Part model, mm, in its own coordinate system. A direction names the side the tool comes from. Coordinates: 2 decimals unless noted, no trailing zeros. Order: outer loops, then holes, each group sorted by start corner. A loop starts at its lowest first (then second) coordinate and runs counter-clockwise, first axis right, second up.
```python
from build123d import *

# Parameters (mm, degrees)
SKETCH_1_R          = 1.6
SKETCH_1_R_2        = 2.1
EXTRUDE_1_DEPTH     = 20
EXTRUDE_2_DEPTH     = 20
SKETCH_3_R          = 1.6
CUT_EXTRUDE_1_DEPTH = 169.07736314
SKETCH_4_R          = 1.6
CUT_EXTRUDE_2_DEPTH = 169.07736314
SKETCH_6_W          = 50
SKETCH_6_H          = 15
SKETCH_6_W_2        = 77.817383139
SKETCH_6_H_2        = 81.542414759
CUT_EXTRUDE_3_DEPTH = 169.07736314
FILLET_1_R          = 2
CUT_EXTRUDE_4_DEPTH = 120.357877938
FILLET_2_R          = 1
SKETCH_8_W          = 15
SKETCH_8_H          = 22
SKETCH_8_H_2        = 25
CUT_EXTRUDE_5_DEPTH = 120.357877938
FILLET_3_R          = 10
FILLET_4_R          = 1
SKETCH_9_W          = 25.911411074
SKETCH_9_H          = 3
EXTRUDE_3_DEPTH     = 20
FILLET_5_R          = 1


with BuildPart() as part:
    # 草图1 → 凸台-拉伸1 (new body)
    with BuildSketch(Plane(origin=(0, 0, 0), x_dir=(1, 0, 0), z_dir=(0, 1, 0))):
        Polygon((-25, 0), (-19, 0), (-19, 165), (19, 165), (19, 0), (25, 0), (25, -15), (-25, -15), align=None)
        with Locations(Location((0, -7.5, 0), (0, 0, 270))):
            Circle(SKETCH_1_R, mode=Mode.SUBTRACT)
        with Locations(Location((20, -7.5, 0), (0, 0, 270))):
            Circle(SKETCH_1_R, mode=Mode.SUBTRACT)
        with Locations(Location((-20, -7.5, 0), (0, 0, 270))):
            Circle(SKETCH_1_R, mode=Mode.SUBTRACT)
        with Locations(Location((-15, 156, 0), (0, 0, 270))):
            Circle(SKETCH_1_R_2, mode=Mode.SUBTRACT)
        with Locations(Location((15, 156, 0), (0, 0, 270))):
            Circle(SKETCH_1_R_2, mode=Mode.SUBTRACT)
    extrude(amount=EXTRUDE_1_DEPTH)

    # 草图2 → 凸台-拉伸2 (add)
    with BuildSketch(Plane(origin=(0, 20, 0), x_dir=(1, 0, 0), z_dir=(0, 1, 0))):
        Polygon((-19, 165), (-25, 0), (-19, 0), align=None)
        Polygon((19, 165), (25, 0), (19, 0), align=None)
    extrude(amount=-EXTRUDE_2_DEPTH)

    # 草图3 → 切除-拉伸1 (cut, through all)
    with BuildSketch(Plane(origin=(0, 20, 0), x_dir=(1, 0, 0), z_dir=(0, 1, 0))):
        with Locations(Location((16, 20, 0), (0, 0, 270))):
            Circle(SKETCH_3_R)
        with Locations(Location((-16, 20, 0), (0, 0, 270))):
            Circle(SKETCH_3_R)
    extrude(amount=-CUT_EXTRUDE_1_DEPTH, mode=Mode.SUBTRACT)

    # 草图4 → 切除-拉伸2 (cut, through all)
    with BuildSketch(Plane(origin=(0, 20, 0), x_dir=(1, 0, 0), z_dir=(0, 1, 0))):
        with Locations(Location((-15, 95, 0), (0, 0, 270))):
            Circle(SKETCH_4_R)
        with Locations(Location((15, 95, 0), (0, 0, 270))):
            Circle(SKETCH_4_R)
    extrude(amount=-CUT_EXTRUDE_2_DEPTH, mode=Mode.SUBTRACT)

    # 草图6 → 切除-拉伸3 (cut, through all)
    with BuildSketch(Plane(origin=(0, 20, 0), x_dir=(1, 0, 0), z_dir=(0, 1, 0))):
        with Locations((0, -7.5)):
            Rectangle(SKETCH_6_W, SKETCH_6_H)
        with Locations((-0.977931814, 155.77120738)):
            Rectangle(SKETCH_6_W_2, SKETCH_6_H_2)
    extrude(amount=-CUT_EXTRUDE_3_DEPTH, mode=Mode.SUBTRACT)

    # 圆角1
    fillet_1_edges = [part.edges().sort_by_distance(p)[0] for p in [
        (20.818181818, 10, -115),
        (25, 10, 0),
        (-25, 10, 0),
        (-20.818181818, 10, -115),
    ]]
    fillet(fillet_1_edges, radius=FILLET_1_R)

    # 草图7 → 切除-拉伸4 (cut, through all)
    with BuildSketch(Plane.XZ):
        Polygon((-13.902481523, -30), (-12.011572432, -82), (12.011572432, -82), (13.902481523, -30), align=None)
    extrude(amount=-CUT_EXTRUDE_4_DEPTH, mode=Mode.SUBTRACT)

    # 圆角2
    fillet_2_edges = [part.edges().sort_by_distance(p)[0] for p in [
        (-12.011572432, 10, -82),
        (-13.902481523, 10, -30),
        (13.902481523, 10, -30),
        (12.011572432, 10, -82),
    ]]
    fillet(fillet_2_edges, radius=FILLET_2_R)

    # 草图8 → 切除-拉伸5 (cut, through all)
    with BuildSketch(Plane(origin=(0, 20, 0), x_dir=(1, 0, 0), z_dir=(0, 1, 0))):
        with Locations((0, 19)):
            Rectangle(SKETCH_8_W, SKETCH_8_H)
        with Locations((0, 94.5)):
            Rectangle(SKETCH_8_W, SKETCH_8_H_2)
    extrude(amount=-CUT_EXTRUDE_5_DEPTH, mode=Mode.SUBTRACT)

    # 圆角3
    fillet_3_edges = [part.edges().sort_by_distance(p)[0] for p in [
        (7.5, 10, -82),
        (-7.5, 10, -82),
        (7.5, 10, -30),
        (-7.5, 10, -30),
    ]]
    fillet(fillet_3_edges, radius=FILLET_3_R)

    # 圆角4
    fillet_4_edges = [part.edges().sort_by_distance(p)[0] for p in [
        (7.5, 10, -8),
        (-7.5, 10, -8),
        (7.5, 10, -107),
        (-7.5, 10, -107),
    ]]
    fillet(fillet_4_edges, radius=FILLET_4_R)

    # 草图9 → 凸台-拉伸3 (add)
    with BuildSketch(Plane(origin=(0, 20, 0), x_dir=(1, 0, 0), z_dir=(0, 1, 0))):
        with Locations((0, 54.536339618)):
            Rectangle(SKETCH_9_W, SKETCH_9_H)
        Polygon((13.064796446, 53.036339618), (12.955705537, 56.036339618), (12.955705537, 53.036339618), align=None)
        Polygon((-12.846614628, 59.036339618), (-12.955705537, 56.036339618), (12.955705537, 56.036339618), (12.846614628, 59.036339618), align=None)
        Polygon((-12.955705537, 53.036339618), (-12.955705537, 56.036339618), (-13.064796446, 53.036339618), align=None)
    extrude(amount=-EXTRUDE_3_DEPTH)

    # 圆角5
    fillet_5_edges = [part.edges().sort_by_distance(p)[0] for p in [
        (-12.846614628, 10, -59.036339618),
        (-13.064796446, 10, -53.036339618),
        (13.064796446, 10, -53.036339618),
        (12.846614628, 10, -59.036339618),
    ]]
    fillet(fillet_5_edges, radius=FILLET_5_R)


solid = part.part
```
(1) Slice it at D-D, the plane y = 6.75. State how many separate pieces and enclosed holes the cut face has, then the cut area to 3 significant figures.
(2) Slice it at A-A, the plane x = 5. Give the cut face in (y, z).
(3) Slice it at C-C, the plane z = -34.5. Give the cut face in (x, y), then the cut area to 3 significant figures.
(4) Probe line 1 (X direction, y = 12.5, z = -20); line 2 (X direction, y = 14, z = -95); line 3 (Z direction, x = -9.5, y = 3.5). List the from-to ranges inside material, lowest first.
(5) Pull direction Z, two halves, no side cores. Call faces 1 (the face through (-20.293, 10.14, -114.425)), 2 (the face through (13.477, 9.86, -41.702)), 3 (the face through (0, 0, -58)): +Z half, -Z half, draft (parallel to the pull), parting line (faces both ways), or undercut.
(6) Tool access for faces 4 (the face through (0, 10, 0)), 5 (the face through (-13.488, 9.86, -41.407)): list every direction of +Z, -Z, +X, -X, +Y, -Y with a clear straight run to the whole face (end or side of a thin tool).
(7) Slice it at B-B, the plane z = -95. Give the cut face in (x, y), then the cut area to 3 significant figures.
(8) Drop flat-ended pins along their axis: pin 1 (2 mm diameter, centred on y = 4, z = -71.5, fed in from +X); pin 2 (3 mm diameter, centred on y = 6, z = -90.5, fed in from -X). Give the stop position or say it passes through.
Here are the results:
1. separate pieces: 1
1. enclosed holes: 6
1. area: 3,290 mm2
2. outline: (0, -115) - (20, -115) - (20, -107) - (0, -107) - close; (0, -59.04) - (20, -59.04) - (20, -53.04) - (0, -53.04) - close; (0, -8) - (20, -8) - (20, 0) - (0, 0) - close
3. outline: (-23.75, 0) - (-13.74, 0) - (-13.74, 20) - (-23.75, 20) - close; (13.74, 0) - (23.75, 0) - (23.75, 20) - (13.74, 20) - close
3. area: 400 mm2
4. line 1: x = -24.27 to -17.6, -14.4 to -7.5, 7.5 to 14.4, 17.6 to 24.27
4. line 2: x = -21.55 to -16.6, -13.4 to -7.5, 7.5 to 13.4, 16.6 to 21.55
4. line 3: z = -115 to -83.91, -59.04 to -53.04, -27.02 to 0
5. face 1: -Z half
5. face 2: undercut
5. face 3: draft
6. face 4: +Z, +X, -X, +Y, -Y
6. face 5: +Y, -Y
7. outline: (-21.55, 0) - (-16.6, 0) - (-16.6, 20) - (-21.55, 20) - close; (-13.4, 0) - (-7.5, 0) - (-7.5, 20) - (-13.4, 20) - close; (7.5, 0) - (13.4, 0) - (13.4, 20) - (7.5, 20) - close; (16.6, 0) - (21.55, 0) - (21.55, 20) - (16.6, 20) - close
7. area: 434 mm2
8. pin 1: stops at x = 22.44
8. pin 2: stops at x = -21.76
